Here's how the part is built. I have some questions about the finished solid (model axes, mm). Face numbers are marked on the shaded views. A direction names the side the tool comes from. Round coordinates to 2 decimals unless told otherwise and drop trailing zeros. Order: outer loops, then holes, each group sorted by start corner. A loop starts at its lowest first (then second) coordinate and runs counter-clockwise, first axis right, second up.
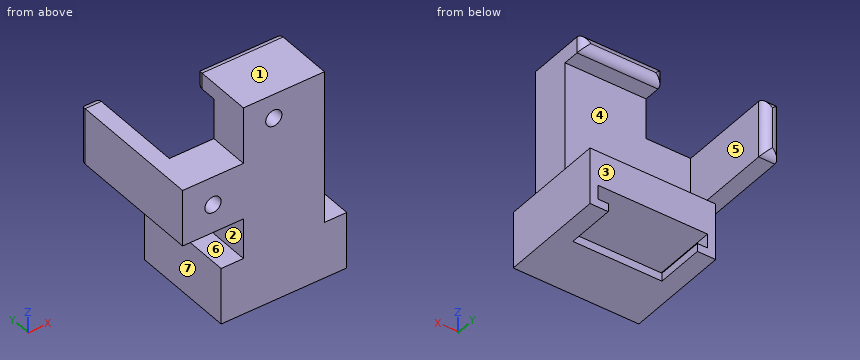
```python
from build123d import *

# Parameters (mm, degrees)
RESSALTO_EXTRUS_O1_DEPTH       = 10
ESBO_O2_W                      = 4
ESBO_O2_H                      = 14
ESBO_O2_W_2                    = 20
ESBO_O2_H_2                    = 4
RESSALTO_EXTRUS_O2_DEPTH       = 25
ESBO_O5_W                      = 20
ESBO_O5_H                      = 42
CORTE_EXTRUS_O1_DEPTH          = 19
FILETE4_R                      = 2
RESSALTO_EXTRUS_O3_DEPTH       = 10
RESSALTO_EXTRUS_O3_DEPTH_BACK  = 4
ESBO_O8_W                      = 31
ESBO_O8_H                      = 4
FURO_DE_DI_METRO_4_0_4_1_D     = 4
FURO_DE_DI_METRO_4_0_4_1_DEPTH = 4
FURO_DE_DI_METRO_4_0_4_1_TIP   = 1.201721238
ESBO_O9_W                      = 27
ESBO_O9_H                      = 3.5
RESSALTO_EXTRUS_O4_DEPTH       = 22
ESBO_O10_W                     = 20
ESBO_O10_H                     = 4
RESSALTO_EXTRUS_O5_DEPTH       = 16
ESBO_O11_W                     = 22
ESBO_O11_H                     = 12
CORTE_EXTRUS_O2_DEPTH          = 2


with BuildPart() as part:
    # Esboço1 → Ressalto-extrusão1 (new body)
    with BuildSketch(Plane(origin=(0, 0, 0), x_dir=(1, 0, 0), z_dir=(0, 1, 0))):
        Polygon((0, 28), (-15, 28), (-15, 14), (0, 14), (0, 0), (20, 0), (20, 42), (0, 42), align=None)
    extrude(amount=RESSALTO_EXTRUS_O1_DEPTH)

    # Esboço2 → Ressalto-extrusão2 (add)
    with BuildSketch(Plane(origin=(0, 10, 0), x_dir=(1, 0, 0), z_dir=(0, 1, 0))):
        with Locations((-13, 21)):
            Rectangle(ESBO_O2_W, ESBO_O2_H)
        with Locations((10, 2)):
            Rectangle(ESBO_O2_W_2, ESBO_O2_H_2)
    extrude(amount=RESSALTO_EXTRUS_O2_DEPTH)

    # Esboço5 → Corte-extrusão1 (cut)
    with BuildSketch(Plane(origin=(0, 35, 0), x_dir=(1, 0, 0), z_dir=(0, 1, 0))):
        with Locations((10, 21)):
            Rectangle(ESBO_O5_W, ESBO_O5_H)
    extrude(amount=-CORTE_EXTRUS_O1_DEPTH, mode=Mode.SUBTRACT)

    # Filete4
    filete4_edges = [part.edges().sort_by_distance(p)[0] for p in [
        (-15, 35, -21),
        (-13, 35, -14),
        (-11, 35, -21),
        (-13, 35, -28),
        (10, 16, -4),
        (20, 16, -2),
        (10, 16, 0),
        (0, 16, -2),
    ]]
    fillet(filete4_edges, radius=FILETE4_R - 0.0001)  # a hair under: the kernel refuses the full size

    # Esboço8 → Ressalto-extrusão3 (add, two sides: drawn at the far end of the back side and taken through both)
    with BuildSketch(Plane(origin=(0, 0, -42), x_dir=(-1, 0, 0), z_dir=(0, 0, -1)).offset(-RESSALTO_EXTRUS_O3_DEPTH_BACK)):
        with Locations((-10, 2)):
            Rectangle(ESBO_O8_W, ESBO_O8_H)
    extrude(amount=RESSALTO_EXTRUS_O3_DEPTH + RESSALTO_EXTRUS_O3_DEPTH_BACK)

    # Furo de diâmetro Ø4.0 (4)1
    with Locations(Plane(origin=(-7.5, 0, -21), x_dir=(0, 0, -1), z_dir=(0, -1, 0))):
        with Locations((0, 0), (-15, 15)):
            Hole(FURO_DE_DI_METRO_4_0_4_1_D / 2, depth=FURO_DE_DI_METRO_4_0_4_1_DEPTH)
            with Locations((0, 0, -(FURO_DE_DI_METRO_4_0_4_1_DEPTH + FURO_DE_DI_METRO_4_0_4_1_TIP / 2))):  # 118° drill point
                Cone(0, FURO_DE_DI_METRO_4_0_4_1_D / 2, FURO_DE_DI_METRO_4_0_4_1_TIP, mode=Mode.SUBTRACT)

    # Esboço9 → Ressalto-extrusão4 (add)
    with BuildSketch(Plane(origin=(0, 4, 0), x_dir=(1, 0, 0), z_dir=(0, 1, 0))):
        Polygon((20, 42), (20, 38), (25.5, 38), (25.5, 52), (-5.5, 52), (-5.5, 38), (0, 38), (0, 42), align=None)
        with Locations((10, 48.25)):
            Rectangle(ESBO_O9_W, ESBO_O9_H, mode=Mode.SUBTRACT)
    extrude(amount=RESSALTO_EXTRUS_O4_DEPTH)

    # Esboço10 → Ressalto-extrusão5 (add)
    with BuildSketch(Plane(origin=(0, 10, 0), x_dir=(1, 0, 0), z_dir=(0, 1, 0))):
        with Locations((10, 40)):
            Rectangle(ESBO_O10_W, ESBO_O10_H)
    extrude(amount=RESSALTO_EXTRUS_O5_DEPTH)

    # Esboço11 → Corte-extrusão2 (cut)
    with BuildSketch(Plane(origin=(0, 0, -52), x_dir=(-1, 0, 0), z_dir=(0, 0, -1))):
        with Locations((-10, 20)):
            Rectangle(ESBO_O11_W, ESBO_O11_H)
    extrude(amount=-CORTE_EXTRUS_O2_DEPTH, mode=Mode.SUBTRACT)


solid = part.part
```
1. If we section it at A-A, the plane y = 3: Write out the boundary of the cut face in (x, z), and give its area (3 significant figures).
Evaluation:
outline: (-15, -28) - (0, -28) - (0, -38) - (-5.5, -38) - (-5.5, -52) - (25.5, -52) - (25.5, -38) - (20, -38) - (20, 0) - (0, 0) - (0, -14) - (-15, -14) - close; hole circle Ø4 at (-7.5, -21); hole circle Ø4 at (7.5, -6)
area: 1,380 mm2
2. I'm going to push flat-ended pins straight in: P1, Ø3, axis at x = 7.5, z = -6, coming from the +Y side; P2, Ø1, axis at x = -2, y = 20.5, coming from the +Z side; P3, Ø4, axis at y = 5, z = -8, coming from the -X side. Where does each tip first touch, or does it pass through?
Evaluation:
P1: stops at y = 10
P2: stops at z = -38
P3: stops at x = 0
3. If we mould it in two halves opening along Z, with no side actions, what happens to the marked faces 1, 2 and 3? For each: released by +Z, released by -Z, zero draft, split by the parting line, or undercut.
Evaluation:
face 1: released by +Z
face 2: undercut
face 3: zero draft
4. On a 3-axis mill with a long thin cutter (end or side, diameter ignored), from which of +Z, -Z, +X, -X, +Y, -Y can I reach the whole of each face in a straight line? I mean the marked faces 4, 5, 6 and 7. Say none if no direction works.
Evaluation:
face 4: +X, +Y
face 5: +Z, -Z, +X, +Y
face 6: +Y
face 7: -Z, -X, +Y, -Y
5. If we section it at D-D, the plane z = -45.5: Write out the boundary of the cut face in (x, y), and give its area (3 significant figures).
Evaluation:
outline: (-5.5, 0) - (25.5, 0) - (25.5, 26) - (-5.5, 26) - close
area: 806 mm2
6. I need wall thicknesses on probe 1 along X at (y, z) = (1.9, -21); probe 2 along Z at (x, y) = (-7.5, 1.2); probe 3 along X at (y, z) = (1, -6). Which ranges of each line are inside material? Lowest first, please.
Evaluation:
probe 1: x = -15 to -9.5, -5.5 to 20
probe 2: z = -28 to -23, -19 to -14
probe 3: x = 0 to 5.5, 9.5 to 20
7. If we section it at B-B, the plane y = 21: Write out the boundary of the cut face in (x, z), and give its area (4 significant figures).
Evaluation:
outline: (-15, -28) - (-11, -28) - (-11, -14) - (-15, -14) - close; (-5.5, -52) - (-1, -52) - (-1, -50) - (-3.5, -50) - (-3.5, -46.5) - (23.5, -46.5) - (23.5, -50) - (21, -50) - (21, -52) - (25.5, -52) - (25.5, -38) - (-5.5, -38) - close
area: 351.5 mm2
